Can you work these out from the model? Positions are in its coordinate system, mm. Coordinates: 2 decimals unless noted, no trailing zeros. Order: outer loops, then holes, each group sorted by start corner. A loop starts at its lowest first (then second) coordinate and runs counter-clockwise, first axis right, second up. Notation, with made-up numbers: M -25.5,70.25 L 21.5,70.25 A30 ccw 21.5,103.25 Z; hole C 22.25,33 d7. An arc over 180 degrees is marked long. Answer as a JSON object with one key per item and string values.
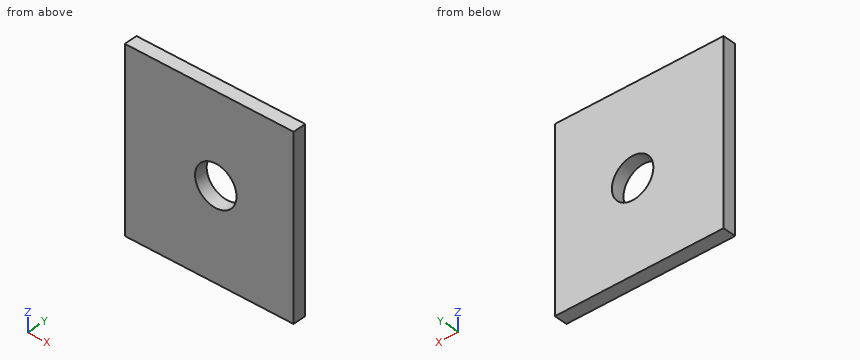
from build123d import *

# Parameters (mm, degrees)
F0_W     = 75
F0_H     = 75
F0_R     = 2.3876
F0_R_2   = 10
F0_W_2   = 6.35
F0_H_2   = 6.35
F1_DEPTH = 6.35


with BuildPart() as f1:
    # F0 (on Front) → F1 (new body)
    with BuildSketch(Plane.XZ):
        Rectangle(F0_W, F0_H)
        with Locations((0, -27.5)):
            Circle(F0_R, mode=Mode.SUBTRACT)
        Circle(F0_R_2, mode=Mode.SUBTRACT)
        with Locations((-40.675, 0)):
            Rectangle(F0_W_2, F0_H)
        with Locations((-40.675, -40.675)):
            Rectangle(F0_W_2, F0_H_2)
        with Locations((0, -40.675)):
            Rectangle(F0_W, F0_H_2)
        Polygon((-37.5, 37.5), (37.5, 37.5), (37.5, 42.5), (-43.85, 42.5), (-43.85, 37.5), align=None)
        with Locations((0, -27.5)):
            Circle(F0_R)
    extrude(amount=F1_DEPTH)


solid = f1.part
Item 1: I want a section at A-A, the plane x = 6. Write out the boundary of the cut face in (y, z), plus the area to 3 significant figures.
Answers follow:
{"outline": "M -6.35,-43.85 L 0,-43.85 L 0,-8 L -6.35,-8 Z; M -6.35,8 L 0,8 L 0,42.5 L -6.35,42.5 Z", "area": "447 mm^2"}
Item 2: I want a section at B-B, the plane z = 0. Write out the boundary of the cut face in (x, y), plus the area to 3 significant figures.
Answers follow:
{"outline": "M -43.85,-6.35 L -10,-6.35 L -10,0 L -43.85,0 Z; M 10,-6.35 L 37.5,-6.35 L 37.5,0 L 10,0 Z", "area": "390 mm^2"}
Item 3: I want a section at C-C, the plane y = -3.75. Write out the boundary of the cut face in (x, z).
Answers follow:
{"outline": "M -43.85,-43.85 L 37.5,-43.85 L 37.5,42.5 L -43.85,42.5 Z; hole C 0,0 d20"}
Item 4: Please list where these lines run through material, in increasing order: line 1 (Z direction, x = 0, y = -2); line 2 (Z direction, x = -4.5, y = -1.25); line 3 (X direction, y = -0.5, z = -8).
Answers follow:
{"line 1": "z = -43.85 to -10, 10 to 42.5", "line 2": "z = -43.85 to -8.93, 8.93 to 42.5", "line 3": "x = -43.85 to -6, 6 to 37.5"}
Item 5: I'm going to push a flat-ended pin straight in: pin 1 (16 mm diameter, centred on x = 0, z = 0, fed in from +Y). Where does the tip first touch, or does it pass through?
Answers follow:
{"pin 1": "passes through"}
